Verification items for the finished model (mm, model axes). A direction names the side the tool comes from. Give positions to 0.01 mm unless a question says otherwise; leave off trailing zeros. Loops run counter-clockwise (first coordinate to the right, second up) from the corner with the lowest first, then second, coordinate; pieces in that order, holes last. Notation, with made-up numbers: (29.25, 11.25) - (57.25, 11.25) arc R18 ccw to (57.25, 27.25) - close; hole circle Ø11 at (42, 11.25). An arc over 180 degrees is marked (long way). Answer in a Markdown table with one row per item.
```python
from build123d import *

# Parameters (mm, degrees)
BOSS_EXTRUDE1_DEPTH = 10
SKETCH2_R           = 1.6
CUT_EXTRUDE1_DEPTH  = 10


with BuildPart() as part:
    # Sketch1 → Boss-Extrude1 (new body)
    with BuildSketch(Plane(origin=(0, 0, 0), x_dir=(0, 0, -1), z_dir=(1, 0, 0))):
        with BuildLine():
            Line((0, 0), (11, 0))
            ThreePointArc((11, 0), (13, 2), (11, 4))
            Line((11, 4), (0, 4))
            ThreePointArc((0, 4), (-6.363961031, 1.363961031), (-9, -5))
            Line((-9, -5), (-9, -10.4))
            ThreePointArc((-9, -10.4), (-7, -12.4), (-5, -10.4))
            Line((-5, -10.4), (-5, -5))
            ThreePointArc((-5, -5), (-3.535533906, -1.464466094), (0, 0))
        make_face()
    extrude(amount=BOSS_EXTRUDE1_DEPTH)

    # Sketch2 → Cut-Extrude1 (cut)
    with BuildSketch(Plane(origin=(0, 4, 0), x_dir=(1, 0, 0), z_dir=(0, 1, 0))):
        with Locations(Location((5, 3.5, 0), (0, 0, 270))):  # turned: the seam where the file's is
            Circle(SKETCH2_R)
    extrude(amount=-CUT_EXTRUDE1_DEPTH, mode=Mode.SUBTRACT)


solid = part.part
```
Q1. Sectioned sample at C-C (y = 0.25). Record the cut outline in (x, z).
Completed:
| item | result |
|---|---|
| outline | (0, -11.97) - (10, -11.97) - (10, 7.31) - (0, 7.31) - close; hole circle Ø3.2 at (5, -3.5) |
Q2. Draft check along X on faces 3 (the face through (3.58, 2.03, -2.76)), 4 (the face through (10, 1, 1)), 5 (the face through (4.9, 0, -5.4)). Enter one of: +X half, -X half, draft (parallel to the pull), parting line (faces both ways), or undercut.
Completed:
| item | result |
|---|---|
| face 3 | undercut |
| face 4 | +X half |
| face 5 | draft |
Q3. Thickness scan on line 1 (X direction, y = 1.35, z = -3.5); line 2 (Y direction, x = 6.5, z = -1.5); line 3 (Z direction, x = 7, y = -9.25). Record the ranges inside material, lowest first.
Completed:
| item | result |
|---|---|
| line 1 | 0 to 3.4, 6.6 to 10 |
| line 2 | 0 to 4 |
| line 3 | 5 to 9 |
Q4. Sectioned sample at A-A (z = -3.5). Record the cut outline in (x, y).
Completed:
| item | result |
|---|---|
| outline | (0, 0) - (3.4, 0) - (3.4, 4) - (0, 4) - close; (6.6, 0) - (10, 0) - (10, 4) - (6.6, 4) - close |
Q5. Tool access check on faces 1 (the face through (5, -8, 5)), 2 (the face through (5, 2, -13)). Record the directions out of +Z, -Z, +X, -X, +Y, -Y that give a thin tool (end or side, any length) a straight path to the whole face; none if there is none.
Completed:
| item | result |
|---|---|
| face 1 | -Z, +X, -X, -Y |
| face 2 | -Z, +X, -X |
Q6. Sectioned sample at D-D (x = 1). Record the cut outline in (y, z), and give its area (3 significant figures).
Completed:
| item | result |
|---|---|
| outline | (-10.4, 5) - (-5, 5) arc R5 cw to (0, 0) - (0, -11) arc R2 ccw to (4, -11) - (4, 0) arc R9 ccw to (-5, 9) - (-10.4, 9) arc R2 ccw to start |
| area | 122 mm^2 |
Q7. Sectioned sample at B-B (x = 5). Record the cut outline in (y, z).
Completed:
| item | result |
|---|---|
| outline | (-10.4, 5) - (-5, 5) arc R5 cw to (0, 0) - (0, -1.9) - (4, -1.9) - (4, 0) arc R9 ccw to (-5, 9) - (-10.4, 9) arc R2 ccw to start; (0, -11) arc R2 ccw to (4, -11) - (4, -5.1) - (0, -5.1) - close |
Q8. Go/stop test with flat-tipped pins: P1, Ø4, axis at x = 5, z = -3.5, coming from the -Y side; P2, Ø1, axis at x = 4.5, y = 1.5, coming from the +Z side; P3, Ø4.5, axis at x = 3, y = -8, coming from the -Z side; P4, Ø3, axis at x = 5, y = 1, coming from the -Z side. Record where each tip stops, or that it passes through.
Completed:
| item | result |
|---|---|
| P1 | y = 0 |
| P2 | z = 6.71 |
| P3 | z = 5 |
| P4 | z = -13 |
